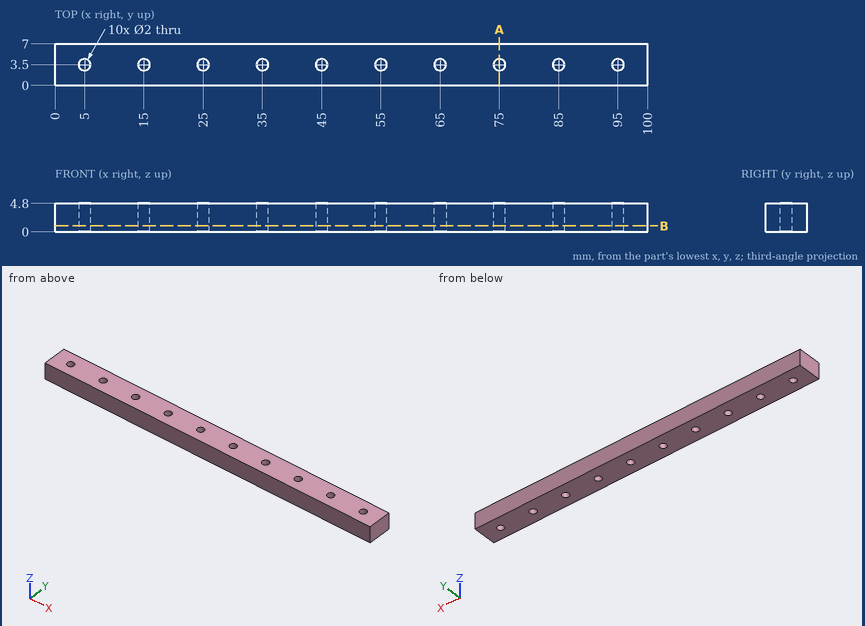
The figure shows three views and two pictorial views of one solid part (mm, origin at its lowest corner). Answer the questions. Coordinates: 2 decimals unless noted, no trailing zeros. Loops run counter-clockwise (first coordinate to the right, second up) from the corner with the lowest first, then second, coordinate; pieces in that order, holes last.
(1) The part is cut by section A-A (x = 75). Determine the outline of the cut face in (y, z), and give its area (3 significant figures).
Solution:
outline: (0, 0) - (2.5, 0) - (2.5, 4.8) - (0, 4.8) - close; (4.5, 0) - (7, 0) - (7, 4.8) - (4.5, 4.8) - close
area: 24.0 mm2
(2) Consider line 1 along Y through (x, z) = (65, 1.05); line 2 along Y through (x, z) = (85.5, 3.3). Determine where each line is inside the solid, lowest interval first.
Solution:
line 1: y = 0 to 2.5, 4.5 to 7
line 2: y = 0 to 2.63, 4.37 to 7
(3) The part is cut by section B-B (z = 1). Count the separate pieces of the cut face and the enclosed holes in it, and give its area (3 significant figures).
Solution:
separate pieces: 1
enclosed holes: 10
area: 669 mm2
(4) Flat-ended cylindrical pins translate along their axes: pin 1 Ø1.6 at (x, y) = (95, 3.5) entering from -Z; pin 2 Ø4 at (x, y) = (57, 4.5) entering from -Z. Find the tip coordinate at first contact, or state that the pin passes through.
Solution:
pin 1: passes through
pin 2: stops at z = 0
